Model file for the job. Use its own axes, mm. A direction names the side the tool comes from. Give positions to 0.01 mm unless a question says otherwise; leave off trailing zeros. Loops run counter-clockwise (first coordinate to the right, second up) from the corner with the lowest first, then second, coordinate; pieces in that order, holes last. Notation, with made-up numbers: (54.25, 16.5) - (86.25, 16.5) arc R24 cw to (86.25, 49.5) - close; hole circle Ø10 at (44, 54). An arc over 180 degrees is marked (long way). Use a Markdown table: item, result.
from build123d import *

# Parameters (mm, degrees)
SKETCH1_R           = 5.5
BOSS_EXTRUDE1_DEPTH = 10


with BuildPart() as part:
    # Sketch1 → Boss-Extrude1 (new body)
    with BuildSketch(Plane.XY):
        with BuildLine():
            Line((9.192533317, -7.713451316), (39.711607161, 28.65776458))
            Line((39.711607161, 28.65776458), (49.357211477, 40.152948176))
            Line((49.357211477, 40.152948176), (135, 40.152948176))
            Line((135, 40.152948176), (135, 64.152948176))
            Line((135, 64.152948176), (38.876588555, 65))
            Line((38.876588555, 65), (-9.192533317, 7.713451316))
            ThreePointArc((-9.192533317, 7.713451316), (-7.713451316, -9.192533317), (9.192533317, -7.713451316))
        make_face()
        Circle(SKETCH1_R, mode=Mode.SUBTRACT)
        with Locations((100, 52.152948176)):
            Circle(SKETCH1_R, mode=Mode.SUBTRACT)
    extrude(amount=BOSS_EXTRUDE1_DEPTH)


solid = part.part
(1) Mould opens along X. For faces 1 (the cylindrical face through (95.635, 48.806, 4.93)), 2 (the flat face through (15.18, 36.76, 4.93)), 3 (the flat face through (56, 44, 10)) say: pulls with the +X half, pulls with the -X half, needs draft (parallel to the pull), parting line crosses it, or undercut.
Computed:
| item | result |
|---|---|
| face 1 | undercut |
| face 2 | pulls with the -X half |
| face 3 | needs draft |
(2) Slice it at B-B, the plane x = 100. Write the cut outline in (y, z), plus the area to 3 significant figures.
Computed:
| item | result |
|---|---|
| outline | (40.15, 0) - (46.65, 0) - (46.65, 10) - (40.15, 10) - close; (57.65, 0) - (64.46, 0) - (64.46, 10) - (57.65, 10) - close |
| area | 133 mm² |
(3) 3-axis set-ups, long thin cutter, end or side, ignore diameter. For faces 4 (the flat face through (92, 40.153, 5)), 5 (the flat face through (135, 52, 5)): which of +Z, -Z, +X, -X, +Y, -Y reach the whole face in a straight line?
Computed:
| item | result |
|---|---|
| face 4 | +Z, -Z, +X, -Y |
| face 5 | +Z, -Z, +X, +Y, -Y |
(4) Drill centre lines: probe 1 along Y at (x, z) = (100, 4.25); probe 2 along Y at (x, z) = (0, 6.25); probe 3 along X at (y, z) = (9, 0.5). Where is each one in solid material? Low to high. Write a range as [from, to].
Computed:
| item | result |
|---|---|
| probe 1 | [40.15, 46.65], [57.65, 64.46] |
| probe 2 | [-12, -5.5], [5.5, 18.67] |
| probe 3 | [-8.11, 23.22] |
(5) Pin check, flat tips, straight feed: P1, Ø9, axis at x = 100, y = 52.15, coming from the -Z side; P2, Ø5, axis at x = 61.5, z = 4, coming from the +Y side; P3, Ø6, axis at y = 38.5, z = 1.5, coming from the -X side; P4, Ø6, axis at y = 32.5, z = 4, coming from the +X side. Stop position of each tip, or through.
Computed:
| item | result |
|---|---|
| P1 | through |
| P2 | y = 64.82 |
| P3 | x = 14.12 |
| P4 | x = 45.45 |
(6) Slice it at D-D, the plane x = 35. Write the cut outline in (y, z).
Computed:
| item | result |
|---|---|
| outline | (23.04, 0) - (60.38, 0) - (60.38, 10) - (23.04, 10) - close |
(7) Slice it at A-A, the plane y = -2. Write the cut outline in (x, z).
Computed:
| item | result |
|---|---|
| outline | (-11.83, 0) - (-5.12, 0) - (-5.12, 10) - (-11.83, 10) - close; (5.12, 0) - (13.99, 0) - (13.99, 10) - (5.12, 10) - close |
(8) Slice it at C-C, the plane z = 5. Write the cut outline in (x, y).
Computed:
| item | result |
|---|---|
| outline | (-9.19, 7.71) arc R12 ccw to (9.19, -7.71) - (49.36, 40.15) - (135, 40.15) - (135, 64.15) - (38.88, 65) - close; hole circle Ø11 at (0, 0); hole circle Ø11 at (100, 52.15) |
